CAD build for the part. Positions are in the model's coordinates, mm. A direction names the side the tool comes from. Give positions to 0.01 mm unless a question says otherwise; leave off trailing zeros. Write each loop counter-clockwise with the first axis right and the second up, starting at its lowest first coordinate (ties: lowest second). Pieces come first, ordered by that corner, then holes. Notation, with made-up numbers: (0.5, 49.5) - (50.5, 49.5) arc R20 cw to (50.5, 62.5) - close; hole circle Ø2 at (32, -25). An arc over 180 degrees is marked (long way). Answer as a JSON object with one key per item and string values.
from build123d import *

# Parameters (mm, degrees)
BOSS_EXTRUDE1_DEPTH = 3.175


with BuildPart() as part:
    # Sketch1 → Boss-Extrude1 (new body)
    with BuildSketch(Plane(origin=(0, 0, 0), x_dir=(1, 0, 0), z_dir=(0, 1, 0))):
        Polygon((-203.6953, 68.834), (-152.8953, 68.834), (-152.8953, 65.659), (-102.0953, 65.659), (-102.0953, 68.834), (102.0953, 68.834), (102.0953, 65.659), (152.8953, 65.659), (152.8953, 68.834), (203.6953, 68.834), (203.6953, -68.834), (152.8953, -68.834), (152.8953, -65.659), (102.0953, -65.659), (102.0953, -68.834), (-102.0953, -68.834), (-102.0953, -65.659), (-152.8953, -65.659), (-152.8953, -68.834), (-203.6953, -68.834), (-206.8703, -68.834), (-206.8703, -43.434), (-203.6953, -43.434), (-203.6953, -18.034), (-206.8703, -18.034), (-206.8703, 18.034), (-203.6953, 18.034), (-203.6953, 43.434), (-206.8703, 43.434), (-206.8703, 68.834), align=None)
        Polygon((-178.464331058, 56.134), (-12.530968942, 56.134), (-95.49765, 7.365766703), align=None, mode=Mode.SUBTRACT)
        Polygon((-190.9953, 48.768233297), (-190.9953, -48.768233297), (-108.028618942, 0), align=None, mode=Mode.SUBTRACT)
        Polygon((-178.464331058, -56.134), (-12.530968942, -56.134), (-95.49765, -7.365766703), align=None, mode=Mode.SUBTRACT)
        Polygon((190.9953, 48.768233297), (190.9953, -48.768233297), (108.028618942, 0), align=None, mode=Mode.SUBTRACT)
        Polygon((6.35, 45.035671291), (6.35, -45.035671291), (82.966681058, 0), align=None, mode=Mode.SUBTRACT)
        Polygon((12.530968942, 56.134), (95.49765, 7.365766703), (178.464331058, 56.134), align=None, mode=Mode.SUBTRACT)
        Polygon((-6.35, 45.035671291), (-6.35, -45.035671291), (-82.966681058, 0), align=None, mode=Mode.SUBTRACT)
        Polygon((12.530968942, -56.134), (178.464331058, -56.134), (95.49765, -7.365766703), align=None, mode=Mode.SUBTRACT)
    extrude(amount=BOSS_EXTRUDE1_DEPTH)


solid = part.part
(1) Flat gauge pins, fed straight in: P1, Ø1, axis at y = 2.5, z = 35.5, coming from the -X side; P2, Ø1, axis at x = 118, y = 1, coming from the -Z side. Where does each tip first touch, or does it go through?
Answer key:
{"P1": "stops at x = -203.7", "P2": "stops at z = -65.66"}
(2) Probe L1, parallel to Z at x = -53, y = 1.8; L2, parallel to Z at x = -85, y = 0.55; L3, parallel to Z at x = -115, y = 2. List the from-to ranges inside material, lowest first. Write a range as [from, to].
Answer key:
{"L1": "z = [-68.83, -56.13], [-32.35, -17.61], [17.61, 32.35], [56.13, 68.83]", "L2": "z = [-68.83, -56.13], [-13.54, 13.54], [56.13, 68.83]", "L3": "z = [-65.66, -56.13], [-18.83, -4.1], [4.1, 18.83], [56.13, 65.66]"}
(3) 3-axis set-ups, long thin cutter, end or side, ignore diameter. For faces 1 (the face through (1, 3.175, -1)), 2 (the face through (148.93, 1.57, -24.04)): which of +Z, -Z, +X, -X, +Y, -Y reach the whole face in a straight line?
Answer key:
{"face 1": "+Z, -Z, +X, -X, +Y", "face 2": "+Y, -Y"}
(4) Saw through at A-A, the plane z = 13. State how many separate pieces and enclosed holes the cut face has, and give its area (3 significant figures).
Answer key:
{"separate pieces": "7", "enclosed holes": "0", "area": "449 mm²"}
(5) Pull direction X, two halves, no side cores. Call faces 3 (the face through (-53.434, 1.565, 32.091)), 4 (the face through (1, 0, -1)): pulls with the +X half, pulls with the -X half, needs draft (parallel to the pull), parting line crosses it, or undercut.
Answer key:
{"face 3": "undercut", "face 4": "needs draft"}
(6) Saw through at B-B, the plane x = 25. Give the cut face in (y, z) (3 decimals), and give its area (3 significant figures).
Answer key:
{"outline": "(0, -68.834) - (3.175, -68.834) - (3.175, -56.134) - (0, -56.134) - close; (0, -48.805) - (3.175, -48.805) - (3.175, -34.073) - (0, -34.073) - close; (0, 34.073) - (3.175, 34.073) - (3.175, 48.805) - (0, 48.805) - close; (0, 56.134) - (3.175, 56.134) - (3.175, 68.834) - (0, 68.834) - close", "area": "174 mm²"}
(7) Saw through at D-D, the plane z = -27. Give the cut face in (x, y) (3 decimals), and give its area (3 significant figures).
Answer key:
{"outline": "(-203.695, 0) - (-190.995, 0) - (-190.995, 3.175) - (-203.695, 3.175) - close; (-153.962, 0) - (-128.9, 0) - (-128.9, 3.175) - (-153.962, 3.175) - close; (-62.095, 0) - (-37.033, 0) - (-37.033, 3.175) - (-62.095, 3.175) - close; (-6.35, 0) - (6.35, 0) - (6.35, 3.175) - (-6.35, 3.175) - close; (37.033, 0) - (62.095, 0) - (62.095, 3.175) - (37.033, 3.175) - close; (128.9, 0) - (153.962, 0) - (153.962, 3.175) - (128.9, 3.175) - close; (190.995, 0) - (203.695, 0) - (203.695, 3.175) - (190.995, 3.175) - close", "area": "439 mm²"}
